Read the model definition and answer for the solid it produces. Units are mm, in the model's axes. A direction names the side the tool comes from. Give positions to 0.01 mm unless a question says otherwise; leave off trailing zeros. Order: outer loops, then holes, each group sorted by start corner. A loop starts at its lowest first (then second) coordinate and runs counter-clockwise, first axis right, second up. Notation, with made-up numbers: (72.25, -29.5) -> (83.25, -29.5) arc R11 cw to (83.25, -12.5) -> close; hole circle Ø1 at (-21.5, 31.25). An arc over 180 degrees is marked (long way). Use one line per item in the form item = value.
Autodesk Inventor part; units mm, degrees
ref_plane "YZ Plane" through (0, 0, 0) normal (1, 0, 0) x (0, 1, 0)
ref_plane "XZ Plane" through (0, 0, 0) normal (0, 1, 0) x (-1, 0, 0)
ref_plane "XY Plane" through (0, 0, 0) normal (0, 0, 1) x (1, 0, 0)
sketch "Sketch1" plane through (-3.78, -1.3516, -16.62) normal (0, 0, 1) x (1, 0, 0)
  line L0 (0, 0) -> (48.2, 0)
  line L1 (48.2, 0) -> (48.2, 4.7063)
  line L2 (48.2, 4.7063) -> (0, 4.7063)
  line L3 (0, 4.7063) -> (0, 0)
extrude "Extrusion1" add sketch "Sketch1" along normal blind 18
sketch "Sketch2" plane through (0, -1.65, -13.93) normal (-1, 0, 0) x (0, 0, 1)
  line L0 (0, 0) -> (5, 0)
  line L1 (5, 0) -> (5, 11.75)
  line L2 (5, 11.75) -> (0, 11.75)
  line L3 (0, 11.75) -> (0, 0)
extrude "Extrusion2" add sketch "Sketch2" along normal blind 2.54
sketch "Sketch3" plane through (5.08, -1.65, -13.93) normal (-1, 0, 0) x (0, 0, 1)
  line L0 (0, 0) -> (5, 0)
  line L1 (5, 0) -> (5, 11.75)
  line L2 (5, 11.75) -> (0, 11.75)
  line L3 (0, 11.75) -> (0, 0)
extrude "Extrusion3" add sketch "Sketch3" along normal blind 2.54
sketch "Sketch4" plane through (2.54, -1.65, -13.93) normal (-1, 0, 0) x (0, 0, 1)
  line L0 (0, 0) -> (5, 0)
  line L1 (5, 0) -> (5, 11.75)
  line L2 (5, 11.75) -> (0, 11.75)
  line L3 (0, 11.75) -> (0, 0)
extrude "Extrusion4" add sketch "Sketch4" along normal blind 2.54
sketch "Sketch5" plane through (-3.5, 1.6, -1.9) normal (1, 0, 0) x (0, 0, -1)
  line L0 (0, 0) -> (6.2, 0)
  line L1 (6.2, 0) -> (6.2, 3.1)
  line L2 (6.2, 3.1) -> (0, 3.1)
  line L3 (0, 3.1) -> (0, 0)
extrude "Extrusion5" add sketch "Sketch5" along normal blind 9.6
sketch "Sketch6" plane through (40, 1.3, -3.62) normal (1, 0, 0) x (0, 0, -1)
  line L0 (0, 0) -> (8, 0)
  line L1 (8, 0) -> (8, 2.95)
  line L2 (8, 2.95) -> (0, 2.95)
  line L3 (0, 2.95) -> (0, 0)
extrude "Extrusion6" add sketch "Sketch6" along normal blind 5.63
sketch "Sketch7" plane through (41.91, 3.25, -13.97) normal (-1, 0, 0) x (0, 0, -1)
  line L0 (0, 0) -> (2.54, 0)
  line L1 (2.54, 0) -> (2.54, 11.75)
  line L2 (2.54, 11.75) -> (0, 11.75)
  line L3 (0, 11.75) -> (0, 0)
extrude "Extrusion7" add sketch "Sketch7" along normal blind 43.18
sketch "Sketch8" plane through (41.91, 3.25, 1.27) normal (-1, 0, 0) x (0, 0, -1)
  line L0 (0, 0) -> (2.54, 0)
  line L1 (2.54, 0) -> (2.54, 11.75)
  line L2 (2.54, 11.75) -> (0, 11.75)
  line L3 (0, 11.75) -> (0, 0)
extrude "Extrusion8" add sketch "Sketch8" along normal blind 43.18
properties part number "ARDUINO MICRO Simplified"
Item 1: The part is cut by section D-D on z = -12.5. Give the vertices of the cut face in (x, y), and give its area (3 significant figures).
Checks:
outline = (-3.78, -1.35) -> (-2.54, -1.35) -> (-2.54, -1.65) -> (5.08, -1.65) -> (5.08, -1.35) -> (44.42, -1.35) -> (44.42, 3.35) -> (5.08, 3.35) -> (5.08, 10.1) -> (-2.54, 10.1) -> (-2.54, 3.35) -> (-3.78, 3.35) -> close
area = 281 mm²
Item 2: Which of the six approach directions +Z, -Z, +X, -X, +Y, -Y give full straight-line access (tool end or side, diameter ignored) to faces 1 (the flat face through (21, -5, -1.27)), 2 (the flat face through (1, 4, -8.1)), 3 (the flat face through (21, -5, 1.27))?
Checks:
face_1 = +X, -X, -Y
face_2 = -X, +Y
face_3 = +Z, +X, -X, -Y
Item 3: The part is cut by section C-C on x = 21.5. Give the vertices of the cut face in (y, z), and give its area (3 significant figures).
Checks:
outline = (-8.5, -16.51) -> (-1.35, -16.51) -> (-1.35, -16.62) -> (3.35, -16.62) -> (3.35, 1.38) -> (-1.35, 1.38) -> (-1.35, 1.27) -> (-8.5, 1.27) -> (-8.5, -1.27) -> (-1.35, -1.27) -> (-1.35, -13.97) -> (-8.5, -13.97) -> close
area = 121 mm²
Item 4: Given pin 1 Ø0.9 at (x, y) = (42, 3.5) entering from +Z; pin 2 Ø5.5 at (x, z) = (31, -11) entering from +Y; pin 3 Ø2 at (x, y) = (28.5, -4) entering from -Z; pin 4 Ø1 at (y, z) = (-2, -9) entering from +X, each flat-ended and moving along its own axis, determine where each tip first touches the part or whether it passes through.
Checks:
pin_1 = 1.38
pin_2 = 3.35
pin_3 = -16.51
pin_4 = 5.08
Item 5: Straight lines are drawn through the part: L1, parallel to Z at x = 16.5, y = -3.75; L2, parallel to X at y = -1.25, z = -8.5; L3, parallel to X at y = 3.5, z = -13. For each, find the intervals that lie inside material, in ascending order. Write a range as from..to.
Checks:
L1 = -16.51..-13.97, -1.27..1.27
L2 = -3.78..44.42
L3 = -2.54..5.08
Item 6: Determine the mould class of faces 4 (the flat face through (-1.27, -5, -15)), 5 (the flat face through (6.1, 4, -5)), 6 (the flat face through (21, -8.5, -15)) for opening direction X: +X half, -X half, draft (parallel to the pull), parting line (faces both ways), or undercut.
Checks:
face_4 = -X half
face_5 = undercut
face_6 = draft
Item 7: The part is cut by section B-B on z = -15. Give the vertices of the cut face in (x, y), and give its area (3 significant figures).
Checks:
outline = (-3.78, -1.35) -> (-1.27, -1.35) -> (-1.27, -8.5) -> (41.91, -8.5) -> (41.91, -1.35) -> (44.42, -1.35) -> (44.42, 3.35) -> (-3.78, 3.35) -> close
area = 536 mm²
Item 8: The part is cut by section A-A on y = -6. Give the vertices of the cut face in (x, z), and give its area (3 significant figures).
Checks:
outline = (-1.27, -16.51) -> (41.91, -16.51) -> (41.91, -13.97) -> (-1.27, -13.97) -> close; (-1.27, -1.27) -> (41.91, -1.27) -> (41.91, 1.27) -> (-1.27, 1.27) -> close
area = 219 mm²
